from build123d import *


with BuildPart() as part:
    # Sweep1: sweep along a path in Sketch2
    with BuildLine(Plane(origin=(0, 0, 0), x_dir=(0, 0, -1), z_dir=(1, 0, 0))) as sweep1_path:
        Line((0, 0), (25.4, 0))
        ThreePointArc((25.4, 0), (109.460186176, 20.143967187), (175.26, 76.2))
    # Sketch1 → Sweep1 (sweep)
    with BuildSketch(Plane.XY):
        with BuildLine():
            Line((-139.7, 0), (139.7, 0))
            ThreePointArc((139.7, 0), (148.680256121, 3.719743879), (152.4, 12.7))
            Line((152.4, 12.7), (149.86, 12.7))
            ThreePointArc((149.86, 12.7), (146.884204897, 5.515795103), (139.7, 2.54))
            Line((139.7, 2.54), (-139.7, 2.54))
            ThreePointArc((-139.7, 2.54), (-146.884204897, 5.515795103), (-149.86, 12.7))
            Line((-149.86, 12.7), (-152.4, 12.7))
            ThreePointArc((-152.4, 12.7), (-148.680256121, 3.719743879), (-139.7, 0))
        make_face()
    sweep(path=sweep1_path.line)


solid = part.part
Part model, mm, in its own coordinate system. A direction names the side the tool comes from. Give positions to 0.01 mm unless a question says otherwise; leave off trailing zeros. Write each loop counter-clockwise with the first axis right and the second up, starting at its lowest first coordinate (ties: lowest second). Pieces come first, ordered by that corner, then holes.
1) Probe L1, parallel to X at y = 12, z = -51; L2, parallel to Y at x = -38, z = -18.5; L3, parallel to X at y = 7, z = -50. List the from-to ranges inside material, lowest first.
Resolved:
L1: x = -152.14 to -149.53, 149.53 to 152.14
L2: y = 0 to 2.54
L3: x = -150.03 to -146.67, 146.67 to 150.03
2) Cut at B-B on z = -12. Write the cut outline in (x, y).
Resolved:
outline: (-152.4, 12.7) arc R12.7 ccw to (-139.7, 0) - (139.7, 0) arc R12.7 ccw to (152.4, 12.7) - (149.86, 12.7) arc R10.16 cw to (139.7, 2.54) - (-139.7, 2.54) arc R10.16 cw to (-149.86, 12.7) - close
3) Pin check, flat tips, straight feed: pin 1 (1 mm diameter, centred on x = 12.5, z = -79, fed in from -Y); pin 2 (3 mm diameter, centred on x = 58.5, z = -88.5, fed in from +Y); pin 3 (2 mm diameter, centred on x = 85, z = -115.5, fed in from -Y). Stop position of each tip, or through.
Resolved:
pin 1: stops at y = 7.76
pin 2: stops at y = 14.33
pin 3: stops at y = 22.8
4) Which spindle directions (+Z, -Z, +X, -X, +Y, -Y) get a long thin tool onto all of the face, cutting with end or side? Do faces 4 (the face through (-1.956, 21.866, -107.233)), 5 (the face through (-2, 0, -13)). Say none if no direction does.
Resolved:
face 4: +Z, +Y
face 5: +Z, -Z, +X, -X, -Y
5) Two-plate mould, pull along X, no slides. Class faces 1 (the face through (-146.805, 5.437, -12.878)), 2 (the face through (151.112, 30.952, -102.688)), 3 (the face through (-148.58, 3.62, -12.88)): released by +X, released by -X, zero draft, split by the parting line, or undercut.
Resolved:
face 1: undercut
face 2: zero draft
face 3: released by -X
6) Cut at A-A on x = -13. Write the cut outline in (y, z).
Resolved:
outline: (0, -25.4) arc R185.46 ccw to (76.2, -175.26) - (77.7, -173.21) arc R182.92 cw to (2.54, -25.4) - (2.54, 0) - (0, 0) - close
